from build123d import *

# Parameters (mm, degrees)
SKETCH1_W           = 42
SKETCH1_H           = 42
SKETCH1_R           = 11.15
SKETCH1_R_2         = 1.85
BOSS_EXTRUDE1_DEPTH = 6
BOSS_EXTRUDE2_DEPTH = 30
CUT_EXTRUDE1_DEPTH  = 87.746757864
SKETCH4_R           = 3
CUT_EXTRUDE2_DEPTH  = 2
CHAMFER1_SIZE       = 4
CHAMFER2_SIZE       = 0.4


with BuildPart() as part:
    # Sketch1 → Boss-Extrude1 (new body)
    with BuildSketch(Plane.XY):
        Rectangle(SKETCH1_W, SKETCH1_H)
        Circle(SKETCH1_R, mode=Mode.SUBTRACT)
        with Locations((15.5, 15.5)):
            Circle(SKETCH1_R_2, mode=Mode.SUBTRACT)
        with Locations((-15.5, 15.5)):
            Circle(SKETCH1_R_2, mode=Mode.SUBTRACT)
        with Locations((-15.5, -15.5)):
            Circle(SKETCH1_R_2, mode=Mode.SUBTRACT)
        with Locations((15.5, -15.5)):
            Circle(SKETCH1_R_2, mode=Mode.SUBTRACT)
    extrude(amount=-BOSS_EXTRUDE1_DEPTH)

    # Sketch2 → Boss-Extrude2 (add)
    with BuildSketch(Plane.XY):
        with BuildLine():
            Line((-35, -60), (55, -60))
            ThreePointArc((55, -60), (33.580179579, -44.353176778), (21, -21))
            Line((21, -21), (-21, -21))
            ThreePointArc((-21, -21), (-24.526439247, -41.746919245), (-35, -60))
        make_face()
    extrude(amount=-BOSS_EXTRUDE2_DEPTH)

    # Sketch3 → Cut-Extrude1 (cut, through all)
    with BuildSketch(Plane(origin=(0, 0, -30), x_dir=(-1, 0, 0), z_dir=(0, 0, -1))):
        with BuildLine():
            Line((-37.363801429, -55), (25.310808042, -55))
            ThreePointArc((25.310808042, -55), (19.013466657, -41.042936644), (16.155813219, -26))
            Line((16.155813219, -26), (-17.317950087, -26))
            ThreePointArc((-17.317950087, -26), (-25.337253654, -41.884976236), (-37.363801429, -55))
        make_face()
    extrude(amount=-CUT_EXTRUDE1_DEPTH, mode=Mode.SUBTRACT)

    # Sketch4 → Cut-Extrude2 (cut)
    with BuildSketch(Plane.XY):
        with Locations((15.5, 15.5)):
            Circle(SKETCH4_R)
        with Locations((15.5, -15.5)):
            Circle(SKETCH4_R)
        with Locations((-15.5, -15.5)):
            Circle(SKETCH4_R)
        with Locations((-15.5, 15.5)):
            Circle(SKETCH4_R)
    extrude(amount=-CUT_EXTRUDE2_DEPTH, mode=Mode.SUBTRACT)

    # Chamfer1
    chamfer1_edges = [part.edges().sort_by_distance(p)[0] for p in [
        (-21, 21, -3),
        (21, 21, -3),
    ]]
    chamfer(chamfer1_edges, length=CHAMFER1_SIZE)

    # Chamfer2
    chamfer2_edges = [part.edges().sort_by_distance(p)[0] for p in [
        (21, -2, 0),
    ]]
    chamfer(chamfer2_edges, length=CHAMFER2_SIZE)
    chamfer2_2_edges = [part.edges().sort_by_distance(p)[0] for p in [
        (18.8, 19.2, 0),
    ]]
    chamfer(chamfer2_2_edges, length=CHAMFER2_SIZE)
    chamfer2_3_edges = [part.edges().sort_by_distance(p)[0] for p in [
        (33.580179579, -44.353176778, 0),
    ]]
    chamfer(chamfer2_3_edges, length=CHAMFER2_SIZE)
    chamfer2_4_edges = [part.edges().sort_by_distance(p)[0] for p in [
        (-0.282842712, 21, 0),
    ]]
    chamfer(chamfer2_4_edges, length=CHAMFER2_SIZE)
    chamfer2_5_edges = [part.edges().sort_by_distance(p)[0] for p in [
        (9.504567043, -60, 0),
    ]]
    chamfer(chamfer2_5_edges, length=CHAMFER2_SIZE)
    chamfer2_6_edges = [part.edges().sort_by_distance(p)[0] for p in [
        (-19.2, 18.8, 0),
    ]]
    chamfer(chamfer2_6_edges, length=CHAMFER2_SIZE)
    chamfer2_7_edges = [part.edges().sort_by_distance(p)[0] for p in [
        (-24.439144818, -41.502075341, 0),
        (-21, -2.282842712, 0),
    ]]
    chamfer(chamfer2_7_edges, length=CHAMFER2_SIZE)
    chamfer2_8_edges = [part.edges().sort_by_distance(p)[0] for p in [
        (6.026496693, -55, 0),
    ]]
    chamfer(chamfer2_8_edges, length=CHAMFER2_SIZE)
    chamfer2_9_edges = [part.edges().sort_by_distance(p)[0] for p in [
        (-19.013466657, -41.042936644, 0),
    ]]
    chamfer(chamfer2_9_edges, length=CHAMFER2_SIZE)
    chamfer2_10_edges = [part.edges().sort_by_distance(p)[0] for p in [
        (25.337253654, -41.884976236, 0),
    ]]
    chamfer(chamfer2_10_edges, length=CHAMFER2_SIZE)
    chamfer2_11_edges = [part.edges().sort_by_distance(p)[0] for p in [
        (0.581068434, -26, 0),
    ]]
    chamfer(chamfer2_11_edges, length=CHAMFER2_SIZE)
    chamfer2_12_edges = [part.edges().sort_by_distance(p)[0] for p in [
        (-18.5, -15.5, 0),
    ]]
    chamfer(chamfer2_12_edges, length=CHAMFER2_SIZE)
    chamfer2_13_edges = [part.edges().sort_by_distance(p)[0] for p in [
        (-11.15, 0, 0),
    ]]
    chamfer(chamfer2_13_edges, length=CHAMFER2_SIZE)
    chamfer2_14_edges = [part.edges().sort_by_distance(p)[0] for p in [
        (-18.5, 15.5, 0),
    ]]
    chamfer(chamfer2_14_edges, length=CHAMFER2_SIZE)
    chamfer2_15_edges = [part.edges().sort_by_distance(p)[0] for p in [
        (12.5, -15.5, 0),
    ]]
    chamfer(chamfer2_15_edges, length=CHAMFER2_SIZE)
    chamfer2_16_edges = [part.edges().sort_by_distance(p)[0] for p in [
        (12.5, 15.5, 0),
    ]]
    chamfer(chamfer2_16_edges, length=CHAMFER2_SIZE)


solid = part.part
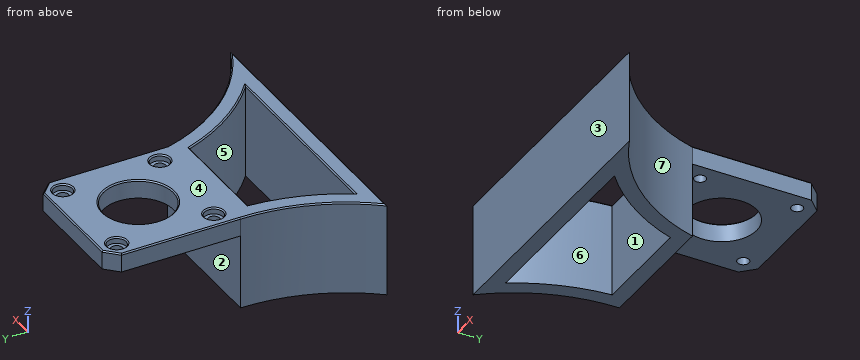
The model under review builds one solid part; all positions refer to its coordinate system, in mm. Face numbers are marked on the shaded views. A direction names the side the tool comes from. Coordinates: 2 decimals unless noted, no trailing zeros. Loops run counter-clockwise (first coordinate to the right, second up) from the corner with the lowest first, then second, coordinate; pieces in that order, holes last. Notation, with made-up numbers: (23, 40.5) -> (64, 40.5) arc R19 ccw to (64, 75.5) -> close; hole circle Ø9 at (14.5, 27.5). An arc over 180 degrees is marked (long way). Use a Markdown table: item, result. Add a question column.
1. Clearance check with flat-ended pins moving along their axes: pin 1 Ø5 at (x, z) = (13.5, -24.5) entering from +Y; pin 2 Ø1.8 at (x, y) = (14.5, -14.5) entering from +Z; pin 3 Ø5 at (x, y) = (15.5, -15.5) entering from -Z. State where each tip first meets the part, or that it passes through.
2. Add section B-B on y = -15.5. Write out the cut boundary in (x, z).
3. To check wall thickness, follow line 1 (Y direction, x = 7, z = -13.5); line 2 (Y direction, x = 0, z = -4); line 3 (X direction, y = 15, z = -3). State the ranges of each line that lie inside material, in increasing order.
4. Draft analysis for pull direction X (two halves, no side actions). For the marked faces 4, 5, 6 and 7, state which applies: pulls with the +X half, pulls with the -X half, needs draft (parallel to the pull), parting line crosses it, or undercut.
5. Machinability: for the marked faces 1, 2 and 3, which of the approach directions +Z, -Z, +X, -X, +Y, -Y give a long, thin tool a straight path to every point of the face, cutting with its end or side? Answer none if there is none.
6. Add section D-D on y = 0. Write out the cut boundary in (x, z).
7. Add section C-C on z = -3.5. Write out the cut boundary in (x, y), plus the area to 3 significant figures.
8. Add section A-A on x = 0. Write out the cut boundary in (y, z), plus the area to 3 significant figures.
Returned:
| question | item | result |
|---|---|---|
| 1 | pin 1 | stops at y = -21 |
| 1 | pin 2 | stops at z = -2 |
| 1 | pin 3 | stops at z = -6 |
| 2 | outline | (-21, -6) -> (-17.35, -6) -> (-17.35, -2) -> (-18.5, -2) -> (-18.5, -0.4) -> (-18.9, 0) -> (-20.6, 0) -> (-21, -0.4) -> close; (-13.65, -6) -> (13.65, -6) -> (13.65, -2) -> (12.5, -2) -> (12.5, -0.4) -> (12.1, 0) -> (-12.1, 0) -> (-12.5, -0.4) -> (-12.5, -2) -> (-13.65, -2) -> close; (17.35, -6) -> (21, -6) -> (21, -0.4) -> (20.6, 0) -> (18.9, 0) -> (18.5, -0.4) -> (18.5, -2) -> (17.35, -2) -> close |
| 3 | line 1 | y = -60 to -55, -26 to -21 |
| 3 | line 2 | y = -60 to -55, -26 to -11.15, 11.15 to 21 |
| 3 | line 3 | x = -21 to -17.28, -13.72 to 13.72, 17.28 to 21 |
| 4 | face 4 | needs draft |
| 4 | face 5 | undercut |
| 4 | face 6 | undercut |
| 4 | face 7 | pulls with the +X half |
| 5 | face 1 | +Z, -Z |
| 5 | face 2 | -Z, +X, -X, +Y |
| 5 | face 3 | +Z, -Z, +X, -X, -Y |
| 6 | outline | (-21, -6) -> (-11.15, -6) -> (-11.15, -0.4) -> (-11.55, 0) -> (-20.6, 0) -> (-21, -0.4) -> close; (11.15, -6) -> (21, -6) -> (21, -0.4) -> (20.6, 0) -> (11.55, 0) -> (11.15, -0.4) -> close |
| 7 | outline | (-35, -60) -> (55, -60) arc R60 cw to (21, -21) -> (21, 17) -> (17, 21) -> (-17, 21) -> (-21, 17) -> (-21, -21) arc R60 cw to start; hole (-25.31, -55) -> (37.36, -55) arc R65 cw to (17.32, -26) -> (-16.16, -26) arc R65 cw to start; hole circle Ø3.7 at (-15.5, -15.5); hole circle Ø3.7 at (-15.5, 15.5); hole circle Ø22.3 at (0, 0); hole circle Ø3.7 at (15.5, -15.5); hole circle Ø3.7 at (15.5, 15.5) |
| 7 | area | 2,280 mm² |
| 8 | outline | (-60, -30) -> (-55, -30) -> (-55, -0.4) -> (-55.4, 0) -> (-59.6, 0) -> (-60, -0.4) -> close; (-26, -30) -> (-21, -30) -> (-21, -6) -> (-11.15, -6) -> (-11.15, -0.4) -> (-11.55, 0) -> (-25.6, 0) -> (-26, -0.4) -> close; (11.15, -6) -> (21, -6) -> (21, -0.4) -> (20.6, 0) -> (11.55, 0) -> (11.15, -0.4) -> close |
| 8 | area | 418 mm² |
